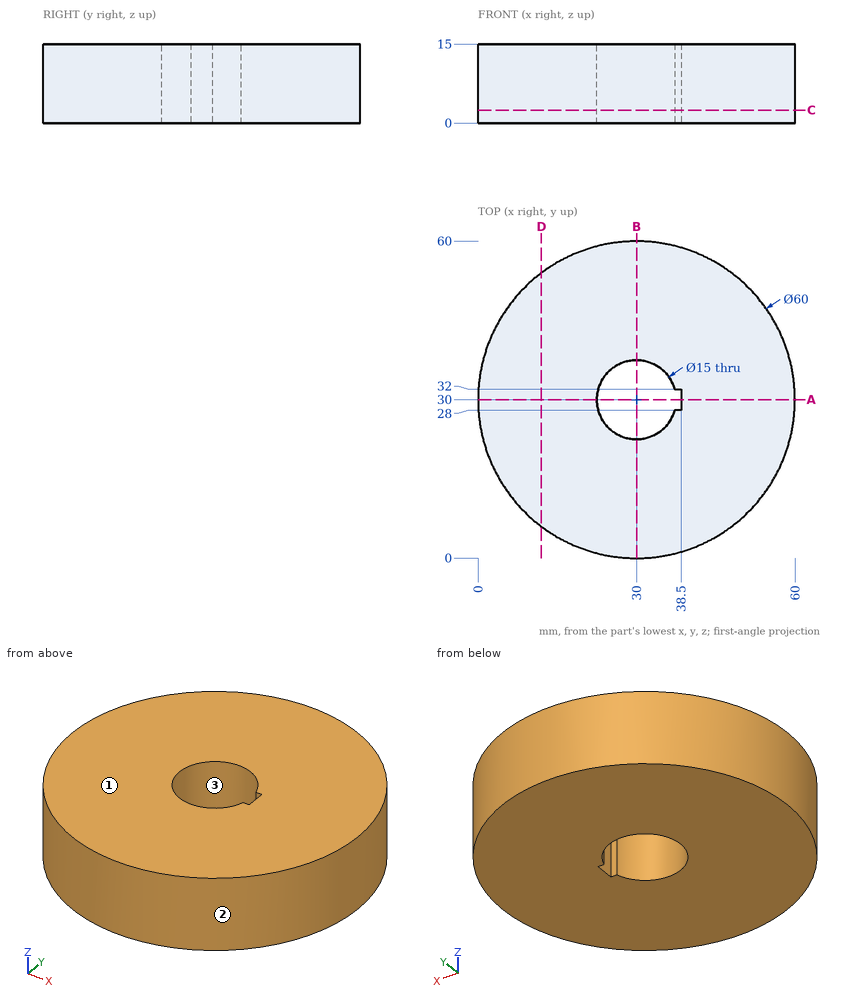
Design review of the part shown in the three views and the two pictorial views. Dimensions are in mm from the part's minimum x, y and z. Round coordinates to 2 decimals unless told otherwise and drop trailing zeros. Order: outer loops, then holes, each group sorted by start corner. A loop starts at its lowest first (then second) coordinate and runs counter-clockwise, first axis right, second up. Notation, with made-up numbers: (-31, -22.5) - (6, -22.5) arc R36 cw to (6, 15.5) - close; hole circle Ø5 at (81.25, 45). An arc over 180 degrees is marked (long way). One line per question, with ' | ' between items.
Item 1: Wall thickness on line 1 (Y direction, x = 25.5, z = 14); line 2 (Y direction, x = 38, z = 8.5); line 3 (X direction, y = 41, z = 9): over which ranges is each line inside the solid? List them lowest first. Write a range as [from, to].
Checks:
line 1: [0.34, 24], [36, 59.66] | line 2: [1.09, 28], [32, 58.91] | line 3: [2.09, 57.91]
Item 2: Take a section at C-C, the plane z = 2.5. Write out the cut boundary in (x, y).
Checks:
outline: circle Ø60 at (30, 30); hole (37.23, 28) - (38.5, 28) - (38.5, 32) - (37.23, 32) arc R7.5 ccw (long way) to start
Item 3: For P1, Ø4, axis at y = 15.5, z = 2, coming from the -X side; P2, Ø4, axis at x = 48, z = 7, coming from the +Y side; P3, Ø8, axis at x = 39.5, z = 3, coming from the -Y side, all flat-tipped, find the tip position at first contact; note any pin that passes through.
Checks:
P1: x = 2.73 | P2: y = 55.38 | P3: y = 0.51
Item 4: Take a section at B-B, the plane x = 30. Write out the cut boundary in (y, z), then the cut area to 3 significant figures.
Checks:
outline: (0, 0) - (22.5, 0) - (22.5, 15) - (0, 15) - close; (37.5, 0) - (60, 0) - (60, 15) - (37.5, 15) - close | area: 675 mm²
Item 5: Draft analysis for pull direction Y (two halves, no side actions). For the marked faces 1, 2 and 3, state which applies: +Y half, -Y half, draft (parallel to the pull), parting line (faces both ways), or undercut.
Checks:
face 1: draft | face 2: parting line | face 3: undercut
Item 6: Take a section at D-D, the plane x = 12. Write out the cut boundary in (y, z), then the cut area to 3 significant figures.
Checks:
outline: (6, 0) - (54, 0) - (54, 15) - (6, 15) - close | area: 720 mm²
Item 7: Take a section at A-A, the plane y = 30. Write out the cut boundary in (x, z).
Checks:
outline: (0, 0) - (22.5, 0) - (22.5, 15) - (0, 15) - close; (38.5, 0) - (60, 0) - (60, 15) - (38.5, 15) - close
